Study the drawing (mm; zero at the part's minimum x, y, z) and answer. A direction names the side the tool comes from. Coordinates: 2 decimals unless noted, no trailing zeros. Write each loop counter-clockwise with the first axis right and the second up, starting at its lowest first coordinate (ties: lowest second). Pieces come first, ordered by that corner, then holes. Notation, with made-up numbers: (64, 10.25) -> (88, 10.25) arc R18 ccw to (88, 23.25) -> close; hole circle Ø6 at (76, 31.25). An arc over 180 degrees is marked (long way). Answer in a Markdown table with one row per item. Add a question column.
Item 1: For a pull along Y with two mould halves and no side action, classify the marked faces 1, 2 and 3 as +Y half, -Y half, draft (parallel to the pull), parting line (faces both ways), or undercut.
Item 2: Section C-C on y = 11 is taken. Write down the section's boundary in (x, z) (1 decimal).
Item 3: Which of the six approach directions +Z, -Z, +X, -X, +Y, -Y give full straight-line access (tool end or side, diameter ignored) to the marked faces 4 and 5?
Item 4: Straight lines are drawn through the part: line 1 (Y direction, x = 14, z = 5.25); line 2 (Y direction, x = 14, z = 9.5); line 3 (X direction, y = 23, z = 9.75). For each, find the intervals that lie inside material, in ascending order. Write a range as from..to.
Item 5: Section A-A on x = 6 is taken. Write down the section's boundary in (y, z) (1 decimal).
Item 6: Section D-D on x = 11 is taken. Write down the section's boundary in (y, z) (1 decimal).
Item 7: Section B-B on z = 12.75 is taken. Write down the section's boundary in (x, y).
Item 8: Given pin 1 Ø6.5 at (y, z) = (12, 11) entering from +X; pin 2 Ø6.5 at (x, z) = (6.5, 11.5) entering from +Y; pin 3 Ø5.5 at (x, y) = (23.17, 22.58) entering from +Z, each flat-ended and moving along its own axis, determine where each tip first touches the part or whether it passes through.
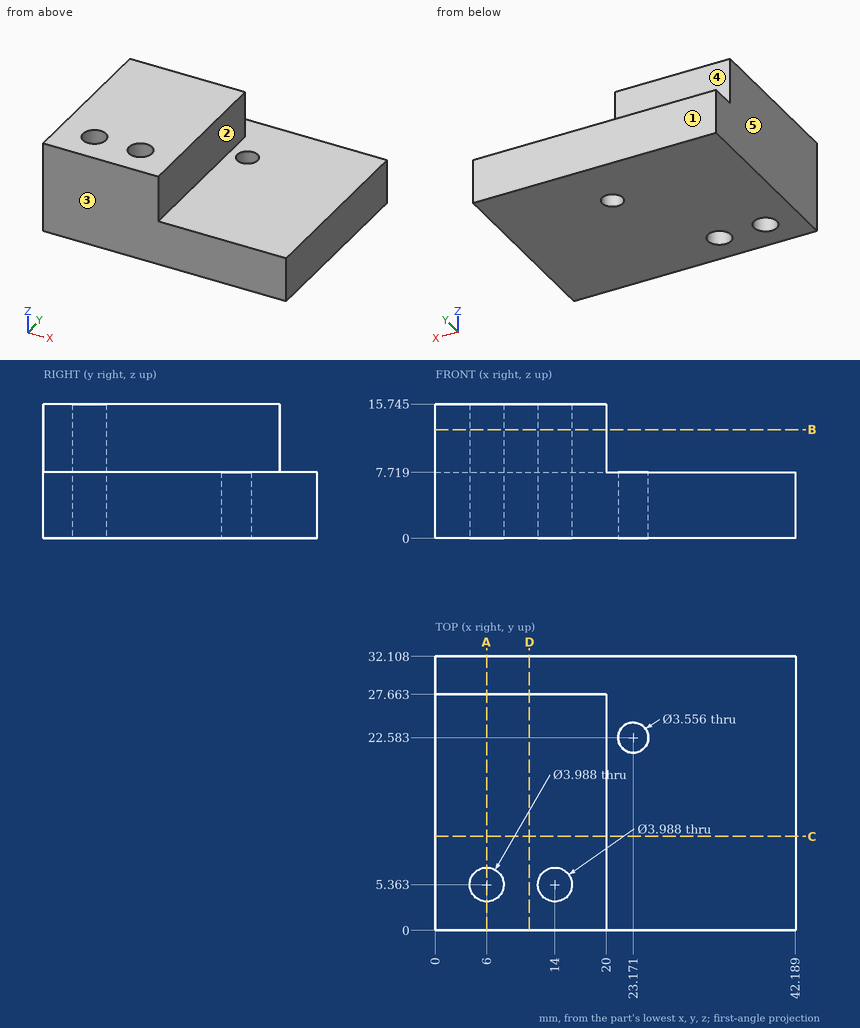
Results below:
| question | item | result |
|---|---|---|
| 1 | face 1 | +Y half |
| 1 | face 2 | draft |
| 1 | face 3 | -Y half |
| 2 | outline | (0, 0) -> (42.2, 0) -> (42.2, 7.7) -> (20, 7.7) -> (20, 15.7) -> (0, 15.7) -> close |
| 3 | face 4 | +Z, +X, -X, +Y |
| 3 | face 5 | +Z, -Z, -X, +Y, -Y |
| 4 | line 1 | y = 0..3.37, 7.36..32.11 |
| 4 | line 2 | y = 0..3.37, 7.36..27.66 |
| 4 | line 3 | x = 0..20 |
| 5 | outline | (0, 0) -> (3.4, 0) -> (3.4, 15.7) -> (0, 15.7) -> close; (7.4, 0) -> (32.1, 0) -> (32.1, 7.7) -> (27.7, 7.7) -> (27.7, 15.7) -> (7.4, 15.7) -> close |
| 6 | outline | (0, 0) -> (32.1, 0) -> (32.1, 7.7) -> (27.7, 7.7) -> (27.7, 15.7) -> (0, 15.7) -> close |
| 7 | outline | (0, 0) -> (20, 0) -> (20, 27.66) -> (0, 27.66) -> close; hole circle Ø3.99 at (6, 5.36); hole circle Ø3.99 at (14, 5.36) |
| 8 | pin 1 | stops at x = 20 |
| 8 | pin 2 | stops at y = 27.66 |
| 8 | pin 3 | stops at z = 7.72 |
